from build123d import *

# Parameters (mm, degrees)
BOSS_EXTRUDE1_DEPTH = 20
SKETCH2_W           = 49.497474684
SKETCH2_H           = 49.497474684
BOSS_EXTRUDE2_DEPTH = 40


with BuildPart() as part:
    # Sketch1 → Boss-Extrude1 (new body)
    with BuildSketch(Plane(origin=(0, 0, 0), x_dir=(1, 0, 0), z_dir=(0, 1, 0))):
        with BuildLine():
            ThreePointArc((-126.808112203, -151.556849545), (-136.118055378, -136.118055378), (-151.556849545, -126.808112203))
            Line((-151.556849545, -126.808112203), (-175.008928344, -150.260191002))
            Line((-175.008928344, -150.260191002), (-150.260191002, -175.008928344))
            Line((-150.260191002, -175.008928344), (-126.808112203, -151.556849545))
        make_face()
        with BuildLine():
            Line((-175.008928344, -150.260191002), (-151.556849545, -126.808112203))
            ThreePointArc((-151.556849545, -126.808112203), (-192.814554121, -184.892545545), (-125.134559673, -162.634559673))
            ThreePointArc((-125.134559673, -162.634559673), (-125.555308196, -157.032853688), (-126.808112203, -151.556849545))
            Line((-126.808112203, -151.556849545), (-150.260191002, -175.008928344))
            Line((-150.260191002, -175.008928344), (-175.008928344, -150.260191002))
        make_face()
        with BuildLine():
            Line((-12.374368671, -12.374368671), (-24.748737342, 0))
            Line((-24.748737342, 0), (-151.556849545, -126.808112203))
            ThreePointArc((-151.556849545, -126.808112203), (-136.118055378, -136.118055378), (-126.808112203, -151.556849545))
            Line((-126.808112203, -151.556849545), (0, -24.748737342))
            Line((0, -24.748737342), (-12.374368671, -12.374368671))
        make_face()
        with BuildLine():
            ThreePointArc((-151.556849545, 126.808112203), (-136.118055378, 136.118055378), (-126.808112203, 151.556849545))
            Line((-126.808112203, 151.556849545), (-150.260191002, 175.008928344))
            Line((-150.260191002, 175.008928344), (-175.008928344, 150.260191002))
            Line((-175.008928344, 150.260191002), (-151.556849545, 126.808112203))
        make_face()
        with BuildLine():
            Line((-150.260191002, 175.008928344), (-126.808112203, 151.556849545))
            ThreePointArc((-126.808112203, 151.556849545), (-125.555308196, 157.032853688), (-125.134559673, 162.634559673))
            ThreePointArc((-125.134559673, 162.634559673), (-192.814554121, 184.892545545), (-151.556849545, 126.808112203))
            Line((-151.556849545, 126.808112203), (-175.008928344, 150.260191002))
            Line((-175.008928344, 150.260191002), (-150.260191002, 175.008928344))
        make_face()
        with BuildLine():
            Line((-24.748737342, 0), (-12.374368671, 12.374368671))
            Line((-12.374368671, 12.374368671), (0, 24.748737342))
            Line((0, 24.748737342), (-126.808112203, 151.556849545))
            ThreePointArc((-126.808112203, 151.556849545), (-136.118055378, 136.118055378), (-151.556849545, 126.808112203))
            Line((-151.556849545, 126.808112203), (-24.748737342, 0))
        make_face()
        with BuildLine():
            Line((126.808112203, 151.556849545), (0, 24.748737342))
            Line((0, 24.748737342), (12.374368671, 12.374368671))
            Line((12.374368671, 12.374368671), (24.748737342, 0))
            Line((24.748737342, 0), (151.556849545, 126.808112203))
            ThreePointArc((151.556849545, 126.808112203), (136.118055378, 136.118055378), (126.808112203, 151.556849545))
        make_face()
        with BuildLine():
            ThreePointArc((200.134559673, 162.634559673), (157.032853688, 199.713811149), (126.808112203, 151.556849545))
            Line((126.808112203, 151.556849545), (150.260191002, 175.008928344))
            Line((150.260191002, 175.008928344), (175.008928344, 150.260191002))
            Line((175.008928344, 150.260191002), (151.556849545, 126.808112203))
            ThreePointArc((151.556849545, 126.808112203), (184.892545545, 132.454565224), (200.134559673, 162.634559673))
        make_face()
        with BuildLine():
            Line((150.260191002, 175.008928344), (126.808112203, 151.556849545))
            ThreePointArc((126.808112203, 151.556849545), (136.118055378, 136.118055378), (151.556849545, 126.808112203))
            Line((151.556849545, 126.808112203), (175.008928344, 150.260191002))
            Line((175.008928344, 150.260191002), (150.260191002, 175.008928344))
        make_face()
        with BuildLine():
            Line((24.748737342, 0), (12.374368671, -12.374368671))
            Line((12.374368671, -12.374368671), (0, -24.748737342))
            Line((0, -24.748737342), (126.808112203, -151.556849545))
            ThreePointArc((126.808112203, -151.556849545), (136.118055378, -136.118055378), (151.556849545, -126.808112203))
            Line((151.556849545, -126.808112203), (24.748737342, 0))
        make_face()
        with BuildLine():
            ThreePointArc((200.134559673, -162.634559673), (184.892545545, -132.454565224), (151.556849545, -126.808112203))
            Line((151.556849545, -126.808112203), (175.008928344, -150.260191002))
            Line((175.008928344, -150.260191002), (150.260191002, -175.008928344))
            Line((150.260191002, -175.008928344), (126.808112203, -151.556849545))
            ThreePointArc((126.808112203, -151.556849545), (157.032853688, -199.713811149), (200.134559673, -162.634559673))
        make_face()
        with BuildLine():
            Line((175.008928344, -150.260191002), (151.556849545, -126.808112203))
            ThreePointArc((151.556849545, -126.808112203), (136.118055378, -136.118055378), (126.808112203, -151.556849545))
            Line((126.808112203, -151.556849545), (150.260191002, -175.008928344))
            Line((150.260191002, -175.008928344), (175.008928344, -150.260191002))
        make_face()
        Polygon((12.374368671, 12.374368671), (0, 0), (12.374368671, -12.374368671), (24.748737342, 0), align=None)
        Polygon((12.374368671, -12.374368671), (0, 0), (-12.374368671, -12.374368671), (0, -24.748737342), align=None)
        Polygon((0, 0), (-12.374368671, 12.374368671), (-24.748737342, 0), align=None)
        Polygon((0, 24.748737342), (-12.374368671, 12.374368671), (0, 0), (12.374368671, 12.374368671), align=None)
        Polygon((-12.374368671, -12.374368671), (0, 0), (-24.748737342, 0), align=None)
    extrude(amount=BOSS_EXTRUDE1_DEPTH)

    # Sketch2 → Boss-Extrude2 (add)
    with BuildSketch(Plane.XZ):
        Rectangle(SKETCH2_W, SKETCH2_H)
    extrude(amount=BOSS_EXTRUDE2_DEPTH)


solid = part.part
Model file for the job. Use its own axes, mm. A direction names the side the tool comes from. Coordinates: 2 decimals unless noted, no trailing zeros. Write each loop counter-clockwise with the first axis right and the second up, starting at its lowest first coordinate (ties: lowest second). Pieces come first, ordered by that corner, then holes. Notation, with made-up numbers: (26, 59) -> (76, 59) arc R22 cw to (76, 84) -> close; hole circle Ø1 at (-28, -1). An arc over 180 degrees is marked (long way). One line per item, written item: value. Start each with the question number.
1) Pull direction X, two halves, no side cores. Call faces 1 (the face through (-64.29, 9.86, 89.04)), 2 (the face through (24.749, -20, 0)), 3 (the face through (0, -20, 24.749)): +X half, -X half, draft (parallel to the pull), parting line (faces both ways), or undercut.
2) Probe probe 1 along X at (y, z) = (-35, -7); probe 2 along X at (y, z) = (10, -83.5); probe 3 along X at (y, z) = (6, 120). List the from-to ranges inside material, lowest first.
3) Flat gauge pins, fed straight in: pin 1 Ø3 at (x, y) = (-6, -5.5) entering from +Z; pin 2 Ø12 at (y, z) = (-20.5, 7) entering from +X; pin 3 Ø20 at (x, y) = (-4.5, -12) entering from -Z. Where does each tip first touch, or does it go through?
4) Slice it at A-A on z = -64. Write the cut outline in (x, y), then the cut area to 3 significant figures.
5) Which spindle directions (+Z, -Z, +X, -X, +Y, -Y) get a long thin tool onto all of the face, cutting with end or side? Do faces 4 (the face through (0, -40, 0)), 5 (the face through (-24.749, -20, 0)), 6 (the face through (0, -20, -24.749)). Say none if no direction does.
6) Slice it at D-D on z = -6. Write the cut outline in (x, y).
7) Slice it at B-B on y = 9. Write the cut outline in (x, z), then the cut area to 3 significant figures.
8) Slice it at C-C on x = 136.5. Write the cut outline in (y, z), then the cut area to 3 significant figures.
Answers follow:
1. face 1: undercut
1. face 2: +X half
1. face 3: draft
2. probe 1: -24.75 to 24.75
2. probe 2: -108.25 to -58.75, 58.75 to 108.25
2. probe 3: -144.75 to -95.25, 95.25 to 144.75
3. pin 1: z = 24.75
3. pin 2: x = 24.75
3. pin 3: z = -24.75
4. outline: (-88.75, 0) -> (-39.25, 0) -> (-39.25, 20) -> (-88.75, 20) -> close; (39.25, 0) -> (88.75, 0) -> (88.75, 20) -> (39.25, 20) -> close
4. area: 1,980 mm2
5. face 4: +Z, -Z, +X, -X, -Y
5. face 5: +Z, -Z, -X, -Y
5. face 6: -Z, +X, -X, -Y
6. outline: (-30.75, 0) -> (-24.75, 0) -> (-24.75, -40) -> (24.75, -40) -> (24.75, 0) -> (30.75, 0) -> (30.75, 20) -> (-30.75, 20) -> close
7. outline: (-151.56, -126.81) arc R37.5 ccw (long way) to (-126.81, -151.56) -> (0, -24.75) -> (126.81, -151.56) arc R37.5 ccw (long way) to (151.56, -126.81) -> (24.75, 0) -> (151.56, 126.81) arc R37.5 ccw (long way) to (126.81, 151.56) -> (0, 24.75) -> (-126.81, 151.56) arc R37.5 ccw (long way) to (-151.56, 126.81) -> (-24.75, 0) -> close
7. area: 43,600 mm2
8. outline: (0, -189.53) -> (20, -189.53) -> (20, -111.75) -> (0, -111.75) -> close; (0, 111.75) -> (20, 111.75) -> (20, 189.53) -> (0, 189.53) -> close
8. area: 3,110 mm2
